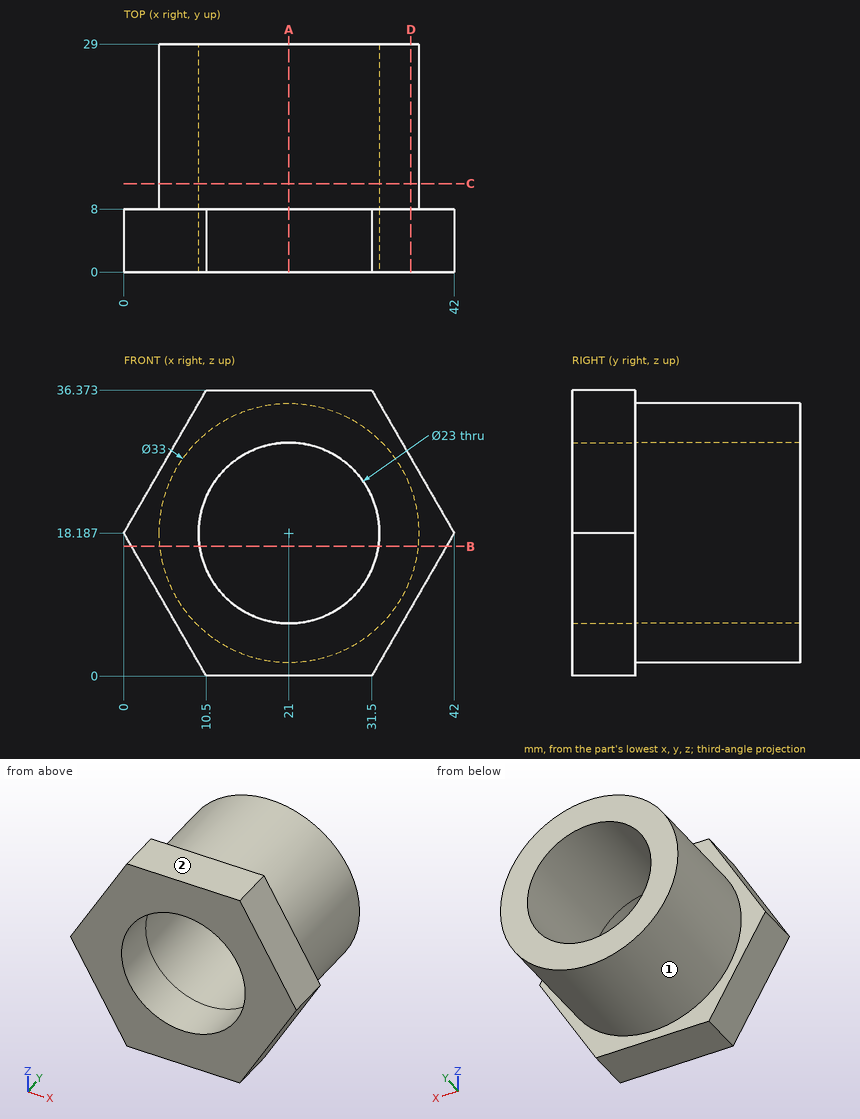
The figure shows three views and two pictorial views of one solid part (mm, origin at its lowest corner). Answer the questions. A direction names the side the tool comes from. Round coordinates to 2 decimals unless told otherwise and drop trailing zeros. Write each loop counter-clockwise with the first axis right and the second up, starting at its lowest first coordinate (ties: lowest second). Pieces come first, ordered by that corner, then holes. Notation, with made-up numbers: (13.5, 23) - (28.5, 23) arc R18 cw to (28.5, 45) - close; hole circle Ø8 at (66, -30). An arc over 180 degrees is marked (long way). Use one line per item in the form item = value. Start each with the question number.
Item 1: A cutting plane is placed at B-B (z = 16.5). Write down the section's boundary in (x, y) (1 decimal), plus the area to 3 significant figures.
Item 2: Flat-ended cylindrical pins translate along their axes: pin 1 Ø1.5 at (y, z) = (6, 11) entering from +X (1 decimal); pin 2 Ø3 at (x, y) = (15.5, 12) entering from -Z; pin 3 Ø20.5 at (x, z) = (21, 18.19) entering from -Y; pin 4 Ø8 at (x, z) = (26.5, 27) entering from +Y. Find the tip coordinate at first contact, or state that the pin passes through.
Item 3: A tool of negligible diameter and unlimited length cuts with its end or side. For the marked faces 1 and 2, from which of +Z, -Z, +X, -X, +Y, -Y can it reach the whole face along a straight path? Write none if from no direction.
Item 4: A cutting plane is placed at D-D (x = 36.5). Write down the section's boundary in (y, z).
Item 5: A cutting plane is placed at A-A (x = 21). Write down the section's boundary in (y, z).
Item 6: A cutting plane is placed at C-C (y = 11.25). Write down the section's boundary in (x, z).
Item 7: Find the intervals of material crossed by line 1 (Z direction, x = 21, y = 12.75); line 2 (Z direction, x = 21, y = 5); line 3 (X direction, y = 9, z = 17), in increasing order. Write a range as [from, to].
The answers:
q1.outline = (1, 0) - (9.6, 0) - (9.6, 29) - (4.6, 29) - (4.6, 8) - (1, 8) - close; (32.4, 0) - (41, 0) - (41, 8) - (37.4, 8) - (37.4, 29) - (32.4, 29) - close
q1.area = 350 mm^2
q2.pin_1 = 38.3
q2.pin_2 = 2.18
q2.pin_3 = through
q2.pin_4 = 29
q3.face_1 = +Y
q3.face_2 = +Z, +X, -X, +Y, -Y
q4.outline = (0, 8.66) - (8, 8.66) - (8, 12.53) - (29, 12.53) - (29, 23.84) - (8, 23.84) - (8, 27.71) - (0, 27.71) - close
q5.outline = (0, 0) - (8, 0) - (8, 1.69) - (29, 1.69) - (29, 6.69) - (0, 6.69) - close; (0, 29.69) - (29, 29.69) - (29, 34.69) - (8, 34.69) - (8, 36.37) - (0, 36.37) - close
q6.outline = circle Ø33 at (21, 18.19); hole circle Ø23 at (21, 18.19)
q7.line_1 = [1.69, 6.69], [29.69, 34.69]
q7.line_2 = [0, 6.69], [29.69, 36.37]
q7.line_3 = [4.54, 9.56], [32.44, 37.46]
